Build history of the part. All positions in model axes, mm. Face numbers are marked on the shaded views. A direction names the side the tool comes from. Round coordinates to 2 decimals unless told otherwise and drop trailing zeros. Write each loop counter-clockwise with the first axis right and the second up, starting at its lowest first coordinate (ties: lowest second). Pieces come first, ordered by that corner, then holes. Notation, with made-up numbers: (-33.75, 1) -> (14.25, 1) arc R15 cw to (14.25, 24) -> close; hole circle Ø7 at (44, -16). An arc over 180 degrees is marked (long way). Answer as CSV lines item,"result".
from build123d import *

# Parameters (mm, degrees)
F1_DEPTH = 19.05
F2_DEPTH = 6.35


with BuildPart() as f1:
    # F0 (on Top) → F1 (new body)
    with BuildSketch(Plane.XY):
        Polygon((50.8, 0), (25.4, 0), (25.4, 25.4), (19.05, 25.4), (19.05, -6.35), (50.8, -6.35), align=None)
    extrude(amount=F1_DEPTH)



with BuildPart() as f1b:
    # F0 (on Top) → F1, piece 2 (new body)
    with BuildSketch(Plane.XY):
        Polygon((50.8, -25.4), (50.8, -19.05), (6.35, -19.05), (6.35, 25.4), (0, 25.4), (0, 0), (0, -25.4), (25.4, -25.4), align=None)
    extrude(amount=F1_DEPTH)


with BuildPart() as f1_1:
    add(f1.part)

    add(f1b.part)  # F2 merges F1b
    # F0 (on Top) → F2 (join)
    with BuildSketch(Plane.XY):
        Polygon((50.8, -19.05), (50.8, -6.35), (19.05, -6.35), (19.05, 25.4), (6.35, 25.4), (6.35, -19.05), align=None)
        Polygon((50.8, 0), (25.4, 0), (25.4, 25.4), (19.05, 25.4), (19.05, -6.35), (50.8, -6.35), align=None)
        Polygon((50.8, -25.4), (50.8, -19.05), (6.35, -19.05), (6.35, 25.4), (0, 25.4), (0, 0), (0, -25.4), (25.4, -25.4), align=None)
    extrude(amount=-F2_DEPTH)


with BuildPart() as f1_2:
    # F3: moved
    add(f1_1.part.moved(Location((0, 0, 6.35))))


solid = f1_2.part
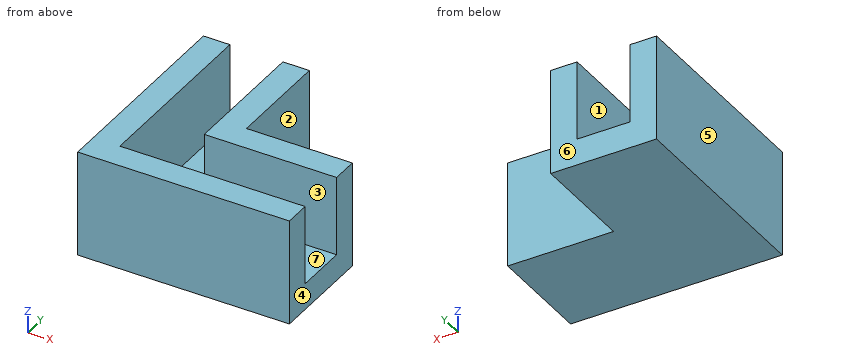
1. Cut at A-A, the plane z = 8.5. Write the cut outline in (x, y).
Results found:
outline,"(0, -25.4) -> (50.8, -25.4) -> (50.8, -19.05) -> (6.35, -19.05) -> (6.35, 25.4) -> (0, 25.4) -> close; (19.05, -6.35) -> (50.8, -6.35) -> (50.8, 0) -> (25.4, 0) -> (25.4, 25.4) -> (19.05, 25.4) -> close"
2. Cut at B-B, the plane x = 47.5. Write the cut outline in (y, z).
Results found:
outline,"(-25.4, 0) -> (0, 0) -> (0, 25.4) -> (-6.35, 25.4) -> (-6.35, 6.35) -> (-19.05, 6.35) -> (-19.05, 25.4) -> (-25.4, 25.4) -> close"
3. Mould opens along X. For the marked faces 4, 5, 6 and 7 say: +X half, -X half, draft (parallel to the pull), parting line (faces both ways), or undercut.
Results found:
face 4,"+X half"
face 5,"-X half"
face 6,"draft"
face 7,"undercut"
4. Which spindle directions (+Z, -Z, +X, -X, +Y, -Y) get a long thin tool onto all of the face, cutting with end or side? Do the marked faces 1, 2 and 3. Say none if no direction does.
Results found:
face 1,"+Z, +Y"
face 2,"+Z, -Z, +X, +Y"
face 3,"+Z, +X"
5. Cut at D-D, the plane y = -12. Write the cut outline in (x, z), then the cut area to 3 significant figures.
Results found:
outline,"(0, 0) -> (50.8, 0) -> (50.8, 6.35) -> (6.35, 6.35) -> (6.35, 25.4) -> (0, 25.4) -> close"
area,"444 mm2"
6. Probe line 1 along Y through (x, z) = (21.5, 7); line 2 along Y through (x, z) = (33, 9.5); line 3 along X through (y, z) = (12.5, 9.5). List the from-to ranges inside material, lowest first.
Results found:
line 1,"y = -25.4 to -19.05, -6.35 to 25.4"
line 2,"y = -25.4 to -19.05, -6.35 to 0"
line 3,"x = 0 to 6.35, 19.05 to 25.4"
7. Cut at C-C, the plane y = 3.5. Write the cut outline in (x, z).
Results found:
outline,"(0, 0) -> (25.4, 0) -> (25.4, 25.4) -> (19.05, 25.4) -> (19.05, 6.35) -> (6.35, 6.35) -> (6.35, 25.4) -> (0, 25.4) -> close"
8. Drop flat-ended pins along their axis: pin 1 Ø15 at (y, z) = (7, 19) entering from +X; pin 2 Ø2 at (x, z) = (34.5, 20.5) entering from +Y; pin 3 Ø1.5 at (x, y) = (38.5, -12.5) entering from +Z; pin 4 Ø12.5 at (y, z) = (7, 12.5) entering from +X. Give the stop position or say it passes through.
Results found:
pin 1,"stops at x = 50.8"
pin 2,"stops at y = 0"
pin 3,"stops at z = 6.35"
pin 4,"stops at x = 25.4"
